Can you work these out from the model? Positions are in its coordinate system, mm. A direction names the side the tool comes from. Round coordinates to 2 decimals unless told otherwise and drop trailing zeros. Order: outer loops, then holes, each group sorted by start corner. A loop starts at its lowest first (then second) coordinate and runs counter-clockwise, first axis right, second up.
Q1. If we section it at C-C (x = -6.5): Please give me the cut outline in (y, z) (3 decimals).
Q2. If we section it at A-A (y = -15.5): Please give me the cut outline in (x, z) (3 decimals).
Q3. We'd pull the mould along X, two halves only. Please class faces 1 (the face through (-11.55, -15.5, -2.5)), 2 (the face through (-2.3, -15.5, -2.6)), 3 (the face through (-5, -18.71, -2.5)), 4 (the face through (-19.1, -6, -3)): pulls with the +X half, pulls with the -X half, needs draft (parallel to the pull), parting line crosses it, or undercut.
Q4. Will these pins go through, and if not, where does the flat tip stop? P1, Ø1.6, axis at x = -4.5, y = -15.5, coming from the +Z side (3 decimals); P2, Ø1, axis at x = -2, y = -13, coming from the -Z side (3 decimals); P3, Ø0.9, axis at y = -17, z = -2.5, coming from the -X side.
Q5. If we section it at D-D (x = -9.25): Please give me the cut outline in (y, z) (3 decimals), plus the area to 3 significant figures.
Q6. For faces 5 (the face through (-5, -15, -2.975)), 6 (the face through (-5, -15, -2.125)), 7 (the face through (-7.55, -15.5, -2.5)), which set-ups out of +Z, -Z, +X, -X, +Y, -Y let a thin tool reach every point of the face, with its end or its side?
Q7. If I drill on line 1 (Y direction, x = -12, z = -3.3); line 2 (Y direction, x = -12.5, z = -4.7); line 3 (Z direction, x = -7, y = -4.75), over which ranges is the centre line in solid material (lowest first)?
Q8. If we section it at B-B (z = -2.5): Please give me the cut outline in (x, y), plus the area to 3 significant figures.
Autodesk Inventor part; units mm, degrees
ref_plane "YZ Plane" through (0, 0, 0) normal (1, 0, 0) x (0, 1, 0)
ref_plane "XZ Plane" through (0, 0, 0) normal (0, 1, 0) x (-1, 0, 0)
ref_plane "XY Plane" through (0, 0, 0) normal (0, 0, 1) x (1, 0, 0)
sketch "Sketch1" plane through (0, 0, 0) normal (0, 1, 0) x (-1, 0, 0)
  line L0 (0, 0) -> (19.1, 0)
  line L1 (19.1, 0) -> (19.1, -5.1)
  line L2 (19.1, -5.1) -> (0, -5.1)
  line L3 (0, -5.1) -> (0, 0)
  dimension "d0" = 19.1
  dimension "d1" = 5.1
extrude "Extrusion1" add sketch "Sketch1" against normal blind 2.29
sketch "Sketch2" plane through (0, 0, 0) normal (1, 0, 0) x (0, 1, 0)
  line L0 (-2.29, -5.1) -> (-2.29, 0)
  line L1 (-2.29, -4.375) -> (-12.29, -4.375) construction
  line L2 (-12.29, -4.375) -> (-12.29, -0.725)
  line L3 (-12.29, -0.725) -> (-2.29, -0.725) construction
  line L4 (-2.29, -0.725) -> (-2.29, -4.375)
  line L5 (0, -5.1) -> (-2.29, -5.1)
  line L6 (-2.29, -4.55) -> (-2.29, -0.55)
  line L7 (-2.29, -4.55) -> (-12.29, -4.375)
  line L8 (-2.29, -0.55) -> (-12.29, -0.725)
  point P0 (0, 0)
  dimension "d5" = 3.65
  dimension "d6" = 0.725
  dimension "d7" = 4
  dimension "d8" = 0.55
  dimension "d19" = 10
extrude "Extrusion2" add sketch "Sketch2" against normal blind 19.1
sketch "Sketch3" plane through (0, -12.29, -4.375) normal (0, -1, 0) x (1, 0, 0)
  line L0 (-16.8, 2.25) -> (-2.3, 2.25) construction
  line L1 (-2.3, 2.25) -> (-2.3, 1.4) construction
  line L2 (-2.3, 1.4) -> (-16.8, 1.4) construction
  line L3 (-16.8, 1.4) -> (-16.8, 2.25) construction
  line L4 (-19.1, 0) -> (-19.1, 3.65)
  line L5 (0, 3.65) -> (-19.1, 3.65)
  line L6 (-16.8, 2.25) -> (-11.55, 2.25)
  line L7 (-11.55, 2.25) -> (-11.55, 1.4)
  line L8 (-11.55, 1.4) -> (-16.8, 1.4)
  line L9 (-16.8, 1.4) -> (-16.8, 2.25)
  line L10 (-2.3, 2.25) -> (-7.55, 2.25)
  line L11 (-7.55, 2.25) -> (-7.55, 1.4)
  line L12 (-7.55, 1.4) -> (-2.3, 1.4)
  line L13 (-2.3, 1.4) -> (-2.3, 2.25)
  point P0 (0, 4.375)
  dimension "d11" = 14.5
  dimension "d12" = 2.3
  dimension "d13" = 0.85
  dimension "d14" = 1.4
  dimension "d15" = 5.25
  dimension "d16" = 5.25
extrude "Extrusion3" add sketch "Sketch3" along normal blind 6.42
properties part number "fuse"
Solution:
1. outline: (-18.71, -2.975) - (-12.29, -2.975) - (-12.29, -4.375) - (-2.29, -4.55) - (-2.29, -5.1) - (0, -5.1) - (0, 0) - (-2.29, 0) - (-2.29, -0.55) - (-12.29, -0.725) - (-12.29, -2.125) - (-18.71, -2.125) - close
2. outline: (-16.8, -2.975) - (-11.55, -2.975) - (-11.55, -2.125) - (-16.8, -2.125) - close; (-7.55, -2.975) - (-2.3, -2.975) - (-2.3, -2.125) - (-7.55, -2.125) - close
3. face 1: undercut
3. face 2: pulls with the +X half
3. face 3: needs draft
3. face 4: pulls with the -X half
4. P1: stops at z = -2.125
4. P2: stops at z = -2.975
4. P3: stops at x = -16.8
5. outline: (-12.29, -4.375) - (-2.29, -4.55) - (-2.29, -5.1) - (0, -5.1) - (0, 0) - (-2.29, 0) - (-2.29, -0.55) - (-12.29, -0.725) - close
5. area: 49.9 mm2
6. face 5: -Z, +X, -X, -Y
6. face 6: +Z, +X, -X, -Y
6. face 7: +Z, -Z, -Y
7. line 1: y = -12.29 to 0
7. line 2: y = -2.29 to 0
7. line 3: z = -4.51 to -0.59
8. outline: (-19.1, -12.29) - (-16.8, -12.29) - (-16.8, -18.71) - (-11.55, -18.71) - (-11.55, -12.29) - (-7.55, -12.29) - (-7.55, -18.71) - (-2.3, -18.71) - (-2.3, -12.29) - (0, -12.29) - (0, 0) - (-19.1, 0) - close
8. area: 302 mm2
